Can you work these out from the model? Positions are in its coordinate system, mm. Face numbers are marked on the shaded views. Give positions to 0.01 mm unless a question says otherwise; leave off trailing zeros. Order: outer loops, then holes, each group sorted by start corner. A loop starts at its lowest first (then second) coordinate and runs counter-clockwise, first axis right, second up. Notation, with made-up numbers: M 49,14 L 71,14 A19 ccw 71,18 Z; hole C -28,-23.75 d3. An arc over 180 degrees is marked long. Use one line per item in the form item = value. Start each with the question number.
1. I want a section at A-A, the plane y = 0. List the corners of the cut face in (x, z) for me.
2. I want a section at B-B, the plane z = 7.5. Count the separate pieces of the cut face and the enclosed holes in it, and give its area (3 significant figures).
3. Will these pins go through, and if not, where does the flat tip stop? P1, Ø3, axis at y = -33.5, z = 7, coming from the -X side; P2, Ø6, axis at x = -35, y = 0, coming from the -Z side; P3, Ø3, axis at x = -0.5, z = 7.5, coming from the -Y side.
4. We'd pull the mould along Y, two halves only. Please class the marked faces 1, 2 and 3: +Y half, -Y half, draft (parallel to the pull), parting line (faces both ways), or undercut.
5. I need wall thicknesses on L1, parallel to Y at x = 0, z = 4.5; L2, parallel to Y at x = -4.5, z = 2.25; L3, parallel to Y at x = 3.5, z = 9.5. Which ranges of each line are inside material? Lowest first, please.
6. I want a section at D-D, the plane y = 23. List the corners of the cut face in (x, z) for me.
```python
from build123d import *

# Parameters (mm, degrees)
SKETCH2_R                    = 45
BOSS_EXTRUDE1_DEPTH          = 10
SKETCH3_R                    = 2.5
CUT_EXTRUDE1_DEPTH           = 65.420493634
SKETCH4_R                    = 5
CUT_EXTRUDE2_DEPTH           = 10
F_1_8_0_125_DIAMETER_HOLE1_D = 3.175


with BuildPart() as part:
    # Sketch2 → Boss-Extrude1 (new body)
    with BuildSketch(Plane.XY):
        Circle(SKETCH2_R)
    extrude(amount=BOSS_EXTRUDE1_DEPTH)

    # Sketch3 → Cut-Extrude1 (cut, through all)
    with BuildSketch(Plane(origin=(0, 0, 0), x_dir=(-1, 0, 0), z_dir=(0, 0, -1))):
        Circle(SKETCH3_R)
    extrude(amount=-CUT_EXTRUDE1_DEPTH, mode=Mode.SUBTRACT)

    # Sketch4 → Cut-Extrude2 (cut)
    with BuildSketch(Plane.XY.offset(10)):
        with Locations((0, 35)):
            Circle(SKETCH4_R)
        with Locations((35, 0)):
            Circle(SKETCH4_R)
        with Locations((0, -35)):
            Circle(SKETCH4_R)
        with Locations((-35, 0)):
            Circle(SKETCH4_R)
    extrude(amount=-CUT_EXTRUDE2_DEPTH, mode=Mode.SUBTRACT)

    # 1/8 (0.125) Diameter Hole1 (through all)
    with Locations(Plane.XY.offset(10)):
        with Locations((0, 23), (23, 0), (0, -23), (-23, 0)):
            Hole(F_1_8_0_125_DIAMETER_HOLE1_D / 2)


solid = part.part
```
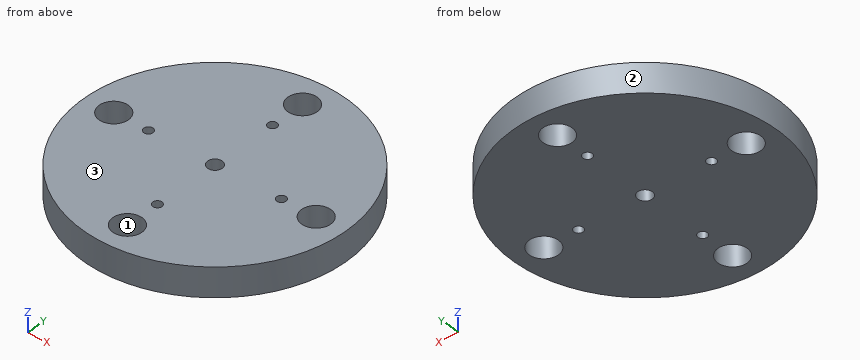
Check result:
q1.outline = M -45,0 L -40,0 L -40,10 L -45,10 Z; M -30,0 L -24.59,0 L -24.59,10 L -30,10 Z; M -21.41,0 L -2.5,0 L -2.5,10 L -21.41,10 Z; M 2.5,0 L 21.41,0 L 21.41,10 L 2.5,10 Z; M 24.59,0 L 30,0 L 30,10 L 24.59,10 Z; M 40,0 L 45,0 L 45,10 L 40,10 Z
q2.separate_pieces = 1
q2.enclosed_holes = 9
q2.area = 6,000 mm2
q3.P1 = -31.64
q3.P2 = through
q3.P3 = -45
q4.face_1 = undercut
q4.face_2 = parting line
q4.face_3 = draft
q5.L1 = -45 to -40, -30 to -24.59, -21.41 to -2.5, 2.5 to 21.41, 24.59 to 30, 40 to 45
q5.L2 = -44.77 to -37.18, -32.82 to 32.82, 37.18 to 44.77
q5.L3 = -44.86 to -38.57, -31.43 to 31.43, 38.57 to 44.86
q6.outline = M -38.68,0 L -1.59,0 L -1.59,10 L -38.68,10 Z; M 1.59,0 L 38.68,0 L 38.68,10 L 1.59,10 Z
